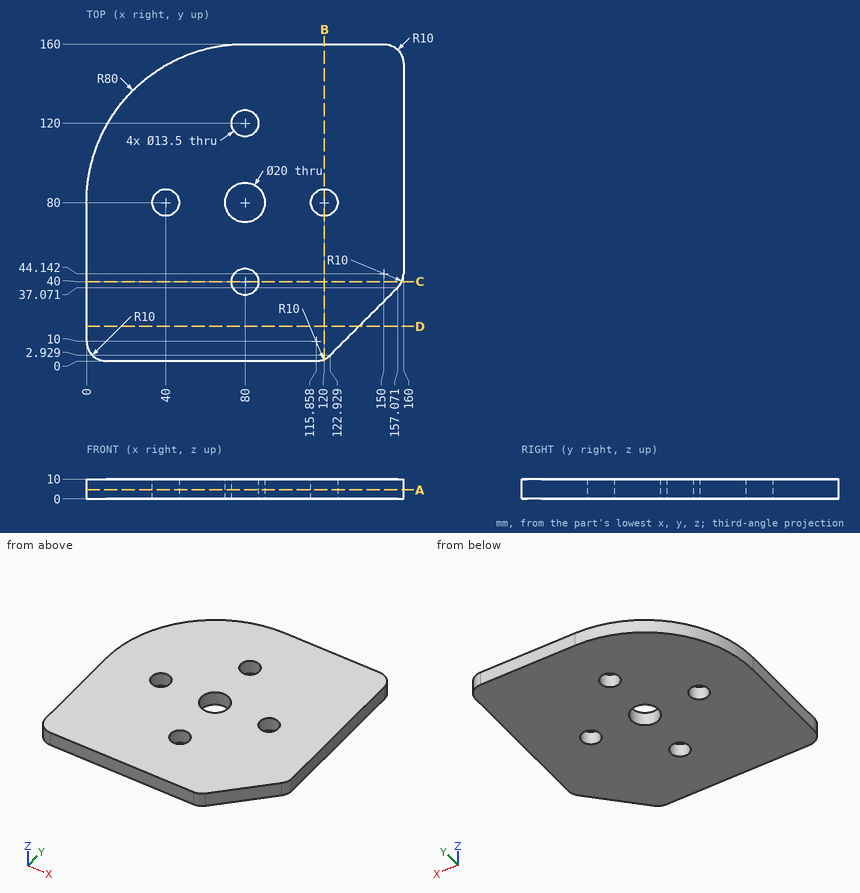
Design review of the part shown in the three views and the two pictorial views. Dimensions are in mm from the part's minimum x, y and z. Round coordinates to 2 decimals unless told otherwise and drop trailing zeros. Loops run counter-clockwise (first coordinate to the right, second up) from the corner with the lowest first, then second, coordinate; pieces in that order, holes last. Notation, with made-up numbers: (40, -2.75) -> (61, -2.75) arc R22 cw to (61, 8.25) -> close; hole circle Ø3 at (39, 36.25). An arc over 180 degrees is marked (long way). Answer as a JSON object with one key per item and string values. Group by question number.
1) For line 1 (Y direction, x = 80, z = 5); line 2 (Y direction, x = 40, z = 7.75); line 3 (Y direction, x = 120, z = 7.75), list the stretches that pass through material, from the lowest coordinate up. Write a range as [from, to].
2) We need section B-B on x = 120. Write out the cut boundary in (y, z).
3) We need section A-A on z = 4.5. Write out the cut boundary in (x, y).
4) We need section C-C on y = 40. Write out the cut boundary in (x, z), then the cut area to 3 significant figures.
5) We need section D-D on y = 17.5. Write out the cut boundary in (x, z).
6) For pin 1 Ø3 at (y, z) = (30, 2.5) entering from +X; pin 2 Ø5 at (y, z) = (106, 6.5) entering from -X; pin 3 Ø4 at (y, z) = (34.5, 3) entering from +X, all flat-tipped, find the tip position at first contact; note any pin that passes through.
Result set:
{
 "1": {"line 1": "[0, 33.25], [46.75, 70], [90, 113.25], [126.75, 160]", "line 2": "[0, 73.25], [86.75, 149.28]", "line 3": "[0.9, 73.25], [86.75, 160]"},
 "2": {"outline": "(0.9, 0) -> (73.25, 0) -> (73.25, 10) -> (0.9, 10) -> close; (86.75, 0) -> (160, 0) -> (160, 10) -> (86.75, 10) -> close"},
 "3": {"outline": "(0, 10) arc R10 ccw to (10, 0) -> (115.86, 0) arc R10 ccw to (122.93, 2.93) -> (157.07, 37.07) arc R10 ccw to (160, 44.14) -> (160, 150) arc R10 ccw to (150, 160) -> (80, 160) arc R80 ccw to (0, 80) -> close; hole circle Ø13.5 at (40, 80); hole circle Ø20 at (80, 80); hole circle Ø13.5 at (80, 40); hole circle Ø13.5 at (80, 120); hole circle Ø13.5 at (120, 80)"},
 "4": {"outline": "(0, 0) -> (73.25, 0) -> (73.25, 10) -> (0, 10) -> close; (86.75, 0) -> (159.1, 0) -> (159.1, 10) -> (86.75, 10) -> close", "area": "1,460 mm²"},
 "5": {"outline": "(0, 0) -> (137.5, 0) -> (137.5, 10) -> (0, 10) -> close"},
 "6": {"pin 1": "x = 151.5", "pin 2": "x = 3.53", "pin 3": "x = 156.5"}
}
